```python
from build123d import *

# Parameters (mm, degrees)
SKETCH1_W           = 4
SKETCH1_H           = 8
SKETCH1_H_2         = 4.5
BOSS_EXTRUDE1_DEPTH = 4
SKETCH1_3_W         = 4
SKETCH1_3_H         = 8
BOSS_EXTRUDE2_DEPTH = 22
SKETCH3_R           = 1.05
CUT_EXTRUDE2_DEPTH  = 15
FILLET1_START       = -0.04496
FILLET1_DEPTH       = 4.04496
FILLET1_START_2     = -4.000000861
FILLET1_2_DEPTH     = 3.955040861
FILLET1_START_3     = 2
FILLET1_3_DEPTH     = 6.5
FILLET1_START_4     = 8.5
FILLET1_4_DEPTH     = 8
FILLET2_R           = 3


with BuildPart() as part:
    # Sketch1 → Boss-Extrude1 (new body)
    # profile 1 of 3: a face of its own
    with BuildSketch(Plane(origin=(0, 0, 0), x_dir=(1, 0, 0), z_dir=(0, 1, 0))):
        with Locations((2, -12.5)):
            Rectangle(SKETCH1_W, SKETCH1_H)
    # profile 2 of 3: a face of its own
    with BuildSketch(Plane(origin=(0, 0, 0), x_dir=(1, 0, 0), z_dir=(0, 1, 0))):
        Polygon((-4, -16.5), (0, -16.5), (0, -8.5), (0, -4), (4, -4), (4, 35.5), (-4, 35.5), align=None)
        with BuildLine():
            ThreePointArc((1.75, 0), (-1.237436867, -1.237436867), (0, 1.75))
            ThreePointArc((0, 1.75), (1.237436867, 1.237436867), (1.75, 0))
        make_face(mode=Mode.SUBTRACT)
        with BuildLine():
            ThreePointArc((1.75, 31), (1.237436867, 29.762563133), (0, 29.25))
            ThreePointArc((0, 29.25), (-1.237436867, 32.237436867), (1.75, 31))
        make_face(mode=Mode.SUBTRACT)
    # profile 3 of 3: a face of its own
    with BuildSketch(Plane(origin=(0, 0, 0), x_dir=(1, 0, 0), z_dir=(0, 1, 0))):
        with Locations((2, -6.25)):
            Rectangle(SKETCH1_W, SKETCH1_H_2)
    extrude(amount=BOSS_EXTRUDE1_DEPTH)

    # Sketch1<3> → Boss-Extrude2 (add)
    with BuildSketch(Plane(origin=(0, 0, 0), x_dir=(1, 0, 0), z_dir=(0, 1, 0))):
        with Locations((2, -12.5)):
            Rectangle(SKETCH1_3_W, SKETCH1_3_H)
    extrude(amount=BOSS_EXTRUDE2_DEPTH)

    # Sketch3 → Cut-Extrude2 (cut)
    with BuildSketch(Plane.ZY):
        with Locations((12.5, 19)):
            Circle(SKETCH3_R)
        with Locations((12.5, 12.5)):
            Circle(SKETCH3_R)
    extrude(amount=-CUT_EXTRUDE2_DEPTH, mode=Mode.SUBTRACT)

    # Fillet1: read off the stored shape, not the designer's step
    # Fillet1 outline → Fillet1 (add)
    with BuildSketch(Plane.YZ.offset(FILLET1_START)):
        with BuildLine():
            ThreePointArc((4, 3.5), (5.464466094, 7.035533906), (9, 8.5))
            Line((9, 8.5), (4, 8.5))
            Line((4, 8.5), (4, 3.5))
        make_face()
    extrude(amount=FILLET1_DEPTH)

    # Fillet1 2 outline → Fillet1 2 (add)
    with BuildSketch(Plane.YZ.offset(FILLET1_START_2)):
        with BuildLine():
            ThreePointArc((4, 3.5), (5.464466094, 7.035533906), (9, 8.5))
            Line((9, 8.5), (4, 8.5))
            Line((4, 8.5), (4, 3.5))
        make_face()
    extrude(amount=FILLET1_2_DEPTH)

    # Fillet1 3 outline → Fillet1 3 (cut)
    with BuildSketch(Plane.XY.offset(FILLET1_START_3)):
        with BuildLine():
            Line((-4.000000861, 10), (-4.000045415, 3.99999073))
            ThreePointArc((-4.000045415, 3.99999073), (-1.127031311, 5.736683874), (0, 8.898979486))
            Line((0, 8.898979486), (0, 10))
            Line((0, 10), (-4.000000861, 10))
        make_face()
    extrude(amount=FILLET1_3_DEPTH, mode=Mode.SUBTRACT)

    # Fillet1 4 outline → Fillet1 4 (add)
    with BuildSketch(Plane.XY.offset(FILLET1_START_4)):
        with BuildLine():
            ThreePointArc((0, 8.898979486), (-1.127031311, 5.736683874), (-4.000045415, 3.99999073))
            Line((-4.000045415, 3.99999073), (0, 4))
            Line((0, 4), (0, 8.898979486))
        make_face()
    extrude(amount=FILLET1_4_DEPTH)

    # Fillet2
    fillet2_edges = [part.edges().sort_by_distance(p)[0] for p in [
        (-4, 2, -35.5),
        (4, 2, -35.5),
    ]]
    fillet(fillet2_edges, radius=FILLET2_R)


solid = part.part
```
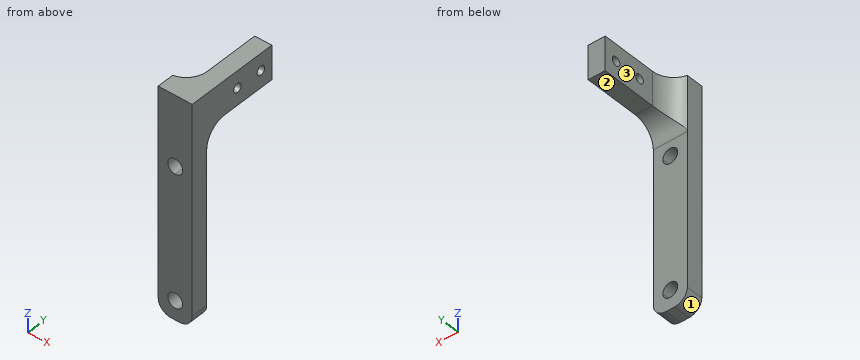
The listing builds one solid part. Answer for the finished solid, in the listing's coordinates (mm). Face numbers are marked on the shaded views. A direction names the side the tool comes from. Coordinates: 2 decimals unless noted, no trailing zeros. Write each loop counter-clockwise with the first axis right and the second up, starting at its lowest first coordinate (ties: lowest second). Pieces come first, ordered by that corner, then holes. Notation, with made-up numbers: (75.25, 16) -> (84.25, 16) arc R32 ccw to (84.25, 52) -> close; hole circle Ø6 at (79, 82). An arc over 180 degrees is marked (long way). Write each question's results on one line, items separated by ' | '. Start each with the question number.
1) A cutting plane is placed at A-A (z = 12.5). Count the separate pieces of the cut face and the enclosed holes in it, then the cut area to 3 significant figures.
2) A cutting plane is placed at B-B (y = 12.5). Determine the outline of the cut face in (x, z).
3) Flat-ended cylindrical pins translate along their axes: pin 1 Ø6.5 at (y, z) = (17.5, 12.5) entering from -X; pin 2 Ø12 at (y, z) = (18, 2) entering from -X; pin 3 Ø4 at (x, y) = (1, 16.5) entering from -Z; pin 4 Ø1.5 at (x, z) = (-3, -19.5) entering from +Y. Find the tip coordinate at first contact, or state that the pin passes through.
4) A cutting plane is placed at C-C (z = -1). Determine the outline of the cut face in (x, y), then the cut area to 3 significant figures.
5) A tool of negligible diameter and unlimited length cuts with its end or side. For the marked faces 1, 2 and 3, from which of +Z, -Z, +X, -X, +Y, -Y can it reach the whole face along a straight path? Write none if from no direction.
6) Straight lines are drawn through the part: probe 1 along X at (y, z) = (3.1, 0); probe 2 along Z at (x, y) = (0, 1.2); probe 3 along Y at (x, z) = (1, -2.5). For each, find the intervals that lie inside material, in ascending order.
7) A cutting plane is placed at D-D (y = 9.5). Determine the outline of the cut face in (x, z), then the cut area to 3 significant figures.
Values follow:
1) separate pieces: 3 | enclosed holes: 0 | area: 92.1 mm²
2) outline: (0, 8.5) -> (4, 8.5) -> (4, 11.45) -> (0, 11.45) -> close; (0, 13.55) -> (4, 13.55) -> (4, 16.5) -> (0, 16.5) -> close
3) pin 1: x = 0 | pin 2: through | pin 3: z = 8.5 | pin 4: y = 4
4) outline: (-4, 0) -> (-1.44, 0) -> (-1.44, 4) -> (-4, 4) -> close; (1.44, 0) -> (4, 0) -> (4, 4) -> (1.44, 4) -> close | area: 20.5 mm²
5) face 1: -Z, -X, +Y, -Y | face 2: -Z, +X, -X, +Y | face 3: +Z, -Z, -X, +Y
6) probe 1: -4 to -1.75, 1.75 to 4 | probe 2: -35.5 to -32.75, -29.25 to -1.75, 1.75 to 16.5 | probe 3: 0 to 4
7) outline: (0, 8.5) -> (4, 8.5) -> (4, 16.5) -> (0, 16.5) -> close | area: 32.0 mm²
